Answer from the drawing. Dimensions are ordinates in mm from the lowest x, y and z of the part. A direction names the side the tool comes from. Round coordinates to 2 decimals unless told otherwise and drop trailing zeros. Write each loop counter-clockwise with the first axis right and the second up, starting at its lowest first coordinate (ties: lowest second). Pieces come first, ordered by that corner, then holes. Notation, with made-up numbers: M 61.25,45 L 108.25,45 A31 cw 108.25,74 Z; hole C -16,-25.5 d10. An arc over 180 degrees is marked long. One line per item, written item: value. Start each with the question number.
(1) Section D-D (y = 10) is taken. Determine the outline of the cut face in (x, z), plus the area to 3 significant figures.
(2) Given P1, Ø6.5, axis at x = 48.4, y = 10, coming from the +Z side; P2, Ø2, axis at y = 17.5, z = 19, coming from the -X side; P3, Ø12, axis at y = 11, z = 19.5, coming from the -X side; P4, Ø10, axis at x = 45, y = 7, coming from the +Z side, each flat-ended and moving along its own axis, determine where each tip first touches the part or whether it passes through.
(3) Consider probe 1 along Z at (x, y) = (16.7, 13.5); probe 2 along X at (y, z) = (10, 9.75) (1 decimal); probe 3 along X at (y, z) = (10, 21.75). Determine where each line is inside the solid, lowest interval first.
(4) For a pull along Z with two mould halves and no side action, classify the marked faces 4, 5, 6 and 7 as released by +Z, released by -Z, zero draft, split by the parting line, or undercut.
(5) Section B-B (z = 23) is taken. Determine the outline of the cut face in (x, y), plus the area to 3 significant figures.
(6) For the marked faces 1, 2 and 3, determine the directions among +Z, -Z, +X, -X, +Y, -Y from which every point of the face is accessible in a straight line to the end or side of a thin tool.
(7) Section C-C (x = 48.4) is taken. Determine the outline of the cut face in (y, z).
(8) Section A-A (x = 31) is taken. Determine the outline of the cut face in (y, z), plus the area to 3 significant figures.
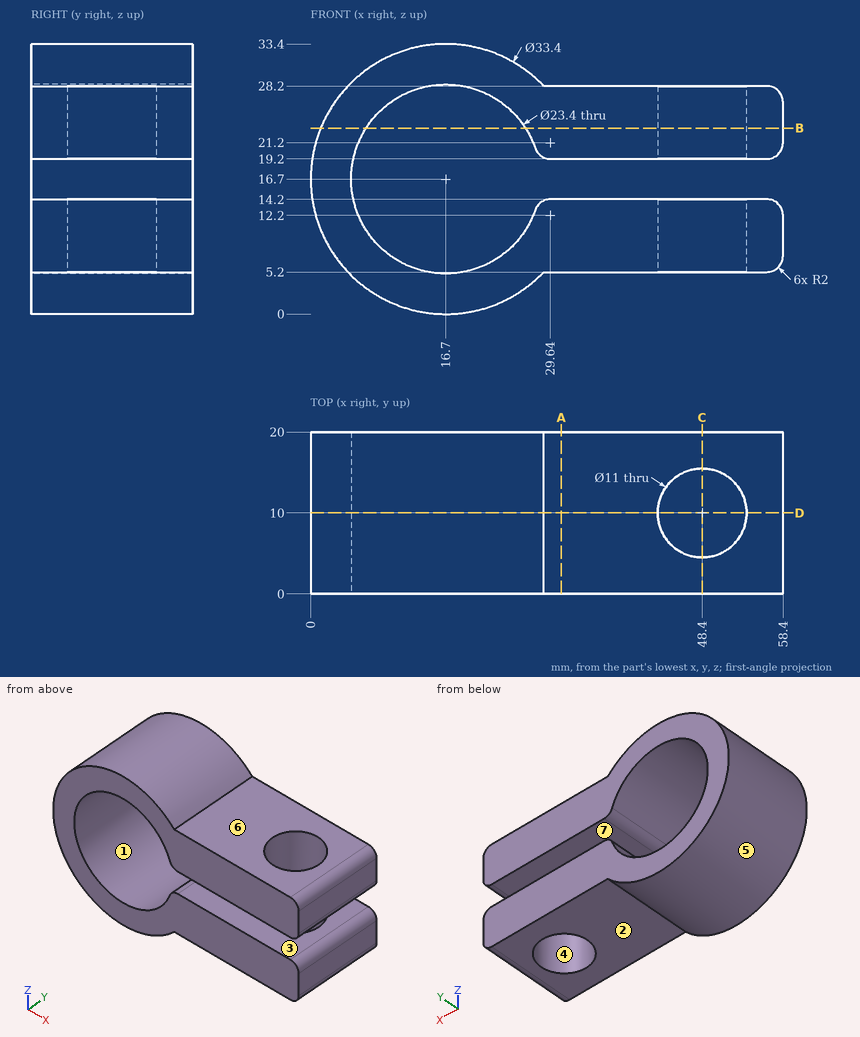
Recorded:
1. outline: M 27.75,12.86 A11.7 cw long 27.75,20.54 A2 ccw 29.64,19.2 L 42.9,19.2 L 42.9,28.2 L 28.81,28.2 A16.7 ccw long 28.81,5.2 L 42.9,5.2 L 42.9,14.2 L 29.64,14.2 A2 ccw Z; M 53.9,5.2 L 56.4,5.2 A2 ccw 58.4,7.2 L 58.4,12.2 A2 ccw 56.4,14.2 L 53.9,14.2 Z; M 53.9,19.2 L 56.4,19.2 A2 ccw 58.4,21.2 L 58.4,26.2 A2 ccw 56.4,28.2 L 53.9,28.2 Z
1. area: 701 mm2
2. P1: passes through
2. P2: stops at x = 0.05
2. P3: stops at x = 0
2. P4: stops at z = 28.2
3. probe 1: z = 0 to 5, 28.4 to 33.4
3. probe 2: x = 1.5 to 7.3, 26.1 to 42.9, 53.9 to 58.4
3. probe 3: x = 0.78 to 6.15, 27.25 to 42.9, 53.9 to 58.4
4. face 4: zero draft
4. face 5: split by the parting line
4. face 6: released by +Z
4. face 7: undercut
5. outline: M 1.23,0 L 6.84,0 L 6.84,20 L 1.23,20 Z; M 26.56,0 L 58.4,0 L 58.4,20 L 26.56,20 Z; hole C 48.4,10 d11
5. area: 654 mm2
6. face 1: +Y, -Y
6. face 2: -Z, +X, +Y, -Y
6. face 3: +X, +Y, -Y
7. outline: M 0,5.2 L 4.5,5.2 L 4.5,14.2 L 0,14.2 Z; M 0,19.2 L 4.5,19.2 L 4.5,28.2 L 0,28.2 Z; M 15.5,5.2 L 20,5.2 L 20,14.2 L 15.5,14.2 Z; M 15.5,19.2 L 20,19.2 L 20,28.2 L 15.5,28.2 Z
8. outline: M 0,5.2 L 20,5.2 L 20,14.2 L 0,14.2 Z; M 0,19.2 L 20,19.2 L 20,28.2 L 0,28.2 Z
8. area: 360 mm2
